Here's how the part is built. I have some questions about the finished solid (model axes, mm). A direction names the side the tool comes from. Coordinates: 2 decimals unless noted, no trailing zeros. Order: outer loops, then holes, each group sorted by start corner. A loop starts at its lowest first (then second) coordinate and runs counter-clockwise, first axis right, second up.
```python
from build123d import *

# Parameters (mm, degrees)
SKETCH1_R           = 3.1
SKETCH1_R_2         = 2.375
BOSS_EXTRUDE1_DEPTH = 4.7625
FILLET1_R           = 0.75
FILLET2_R           = 1.5
CUT_EXTRUDE1_DEPTH  = 5.7625
SKETCH3_R           = 6.883378158
SKETCH3_R_2         = 4.027347077
SKETCH3_R_3         = 2.023736097
SKETCH3_R_4         = 5.007052744
SKETCH3_R_5         = 2.371370049
CUT_EXTRUDE2_DEPTH  = 5.7625


with BuildPart() as part:
    # Sketch1 → Boss-Extrude1 (new body)
    with BuildSketch(Plane(origin=(0, 0, 0), x_dir=(1, 0, 0), z_dir=(0, 1, 0))):
        with BuildLine():
            Line((-2.686438344, 87.958985039), (-0.5, 79.998437485))
            Line((-0.5, 79.998437485), (4.614887054, 86.172076174))
            ThreePointArc((4.614887054, 86.172076174), (5.661584951, 91.971127787), (1.242075777, 95.868885443))
            Line((1.242075777, 95.868885443), (-49.229512188, 106.596952642))
            ThreePointArc((-49.229512188, 106.596952642), (-50.017902784, 107.489183117), (-49.393900435, 108.503212713))
            ThreePointArc((-49.393900435, 108.503212713), (-45.503212713, 117.606099565), (-54.606099565, 121.496787287))
            ThreePointArc((-54.606099565, 121.496787287), (-59.359536161, 118.443728777), (-62.646533103, 113.84895165))
            Line((-62.646533103, 113.84895165), (-94.564318795, 44.533048109))
            ThreePointArc((-94.564318795, 44.533048109), (-94.590381999, 39.571360115), (-90.871592859, 36.28660223))
            Line((-90.871592859, 36.28660223), (-82.579358815, 33.74664323))
            Line((-82.579358815, 33.74664323), (-85.704155619, 43.38101369))
            ThreePointArc((-85.704155619, 43.38101369), (-70.503668965, 59.408545121), (-51.790728612, 71.145768882))
            ThreePointArc((-51.790728612, 71.145768882), (-28.506341212, 83.254960878), (-2.686438344, 87.958985039))
        make_face()
        with Locations((-57, 80)):
            Circle(SKETCH1_R, mode=Mode.SUBTRACT)
        with Locations((-52, 115)):
            Circle(SKETCH1_R_2, mode=Mode.SUBTRACT)
    extrude(amount=BOSS_EXTRUDE1_DEPTH)

    # Fillet1
    fillet1_edges = [part.edges().sort_by_distance(p)[0] for p in [
        (-82.579358815, 2.38125, -33.74664323),
        (-0.5, 2.38125, -79.998437485),
    ]]
    fillet(fillet1_edges, radius=FILLET1_R)

    # Fillet2
    fillet2_edges = [part.edges().sort_by_distance(p)[0] for p in [
        (-85.704155619, 2.38125, -43.38101369),
        (-2.686438344, 2.38125, -87.958985039),
    ]]
    fillet(fillet2_edges, radius=FILLET2_R)

    # Sketch2 → Cut-Extrude1 (cut, through all)
    with BuildSketch(Plane(origin=(0, 4.7625, 0), x_dir=(1, 0, 0), z_dir=(0, 1, 0))):
        with BuildLine():
            Line((-83.074868749, 35.237466844), (-86.244425002, 41.206104458))
            ThreePointArc((-86.244425002, 41.206104458), (-86.416137903, 42.011960676), (-86.136312483, 42.786936353))
            ThreePointArc((-86.136312483, 42.786936353), (-85.690987138, 43.398953447), (-85.240414354, 44.007117694))
            Line((-85.240414354, 44.007117694), (-83.023850343, 35.117099074))
            ThreePointArc((-83.023850343, 35.117099074), (-83.046731861, 35.178396715), (-83.074868749, 35.237466844))
        make_face()
    extrude(amount=-CUT_EXTRUDE1_DEPTH, mode=Mode.SUBTRACT)

    # Sketch3 → Cut-Extrude2 (cut, through all)
    with BuildSketch(Plane(origin=(0, 4.7625, 0), x_dir=(1, 0, 0), z_dir=(0, 1, 0))):
        with Locations((-44.625253906, 92.935332876)):
            Circle(SKETCH3_R)
        with Locations((-28.753871163, 93.427681096)):
            Circle(SKETCH3_R_2)
        with Locations((-17.332089479, 93.427681096)):
            Circle(SKETCH3_R_3)
        with Locations((-70.829162085, 71.852500768)):
            Circle(SKETCH3_R_4)
        with Locations((-78.10497123, 62.687125815)):
            Circle(SKETCH3_R_5)
    extrude(amount=-CUT_EXTRUDE2_DEPTH, mode=Mode.SUBTRACT)


solid = part.part
```
Q1. If we section it at A-A on x = -42.5: Write out the boundary of the cut face in (y, z), then the cut area to 3 significant figures.
Q2. If we section it at D-D on x = -7: Write out the boundary of the cut face in (y, z), then the cut area to 3 significant figures.
Q3. For faces 4 (the flat face through (-84.637, 2.415, -38.18)), 5 (the cylindrical face through (-29.41, 2.35, -82.94)), 6 (the cylindrical face through (-94.62, 2.35, -39.64)), which set-ups out of +Z, -Z, +X, -X, +Y, -Y let a thin tool reach every point of the face, with its end or its side?
Q4. I need wall thicknesses on L1, parallel to X at y = 4.05, z = -95; L2, parallel to Z at x = -50.5, y = 4.5; L3, parallel to Z at x = -39.5, y = 4.3. Which ranges of each line are inside material? Lowest first, please.
Q5. We'd pull the mould along Z, two halves only. Please class faces 1 (the flat face through (-87.46, 2.35, -35.24)), 2 (the cylindrical face through (-50.72, 2.35, -117)), 3 (the cylindrical face through (5.69, 2.35, -91.89)): pulls with the +Z half, pulls with the -Z half, needs draft (parallel to the pull), parting line crosses it, or undercut.
Q6. If we section it at B-B on y = 3.9: Give the number of separate pieces and of enclosed holes in the cut face, then the cut area to 3 significant figures.
Q7. If we section it at C-C on z = -115: Write out the boundary of the cut face in (x, y) (1 decimal).
Q8. Will these pins go through, and if not, where does the flat tip stop? pin 1 (1 mm diameter, centred on y = 3, z = -82.5, fed in from +X); pin 2 (2 mm diameter, centred on x = -72.5, y = 4, fed in from -Z); pin 3 (9 mm diameter, centred on x = -70.83, z = -71.85, fed in from +Y).
Reply:
1. outline: (0, -105.17) - (4.76, -105.17) - (4.76, -99.48) - (0, -99.48) - close; (0, -86.39) - (4.76, -86.39) - (4.76, -77.06) - (0, -77.06) - close
1. area: 71.5 mm2
2. outline: (0, -97.62) - (4.76, -97.62) - (4.76, -87.72) - (0, -87.72) - close
2. area: 47.1 mm2
3. face 4: +X, +Y, -Y
3. face 5: +Z, +Y, -Y
3. face 6: -X, +Y, -Y
4. L1: x = -71.33 to -51.19, -38.06 to -32.46, -25.05 to -18.61, -16.06 to 3.31
4. L2: z = -121.84 to -116.84, -113.16 to -96.52, -89.35 to -72.07
4. L3: z = -104.53 to -97.53, -88.34 to -78.64
5. face 1: pulls with the +Z half
5. face 2: undercut
5. face 3: parting line crosses it
6. separate pieces: 1
6. enclosed holes: 7
6. area: 2,270 mm2
7. outline: (-62.1, 0) - (-54.4, 0) - (-54.4, 4.8) - (-62.1, 4.8) - close; (-49.6, 0) - (-45, 0) - (-45, 4.8) - (-49.6, 4.8) - close
8. pin 1: stops at x = 1.99
8. pin 2: stops at z = -94.62
8. pin 3: passes through
